Verification items for the finished model (mm, model axes). Face numbers are marked on the shaded views. A direction names the side the tool comes from. Give positions to 0.01 mm unless a question says otherwise; leave off trailing zeros. Order: outer loops, then holes, each group sorted by start corner. A loop starts at its lowest first (then second) coordinate and runs counter-clockwise, first axis right, second up.
from build123d import *

# Parameters (mm, degrees)
SKETCH1_W           = 30
SKETCH1_H           = 30
BOSS_EXTRUDE1_DEPTH = 7
SHELL1_T            = -1
SKETCH2_W           = 30
SKETCH2_H           = 7
BOSS_EXTRUDE2_DEPTH = 30
SKETCH3_W           = 30
SKETCH3_H           = 7
BOSS_EXTRUDE3_DEPTH = 30
SKETCH5_W           = 5
SKETCH5_H           = 23
BOSS_EXTRUDE4_DEPTH = 5
CUT_EXTRUDE6_DEPTH  = 23
SKETCH12_W          = 7.071067812
SKETCH12_H          = 23
BOSS_EXTRUDE6_DEPTH = 30
CUT_EXTRUDE7_DEPTH  = 22
CUT_EXTRUDE8_DEPTH  = 22
SHELL2_START        = 24
SHELL2_DEPTH        = 5
SHELL2_START_2      = 23
SHELL2_2_DEPTH      = 1
SHELL2_START_3      = 1
SHELL2_3_DEPTH      = 22
BOSS_EXTRUDE7_DEPTH = 1
BOSS_EXTRUDE8_DEPTH = 23
CUT_EXTRUDE10_DEPTH = 1
CUT_EXTRUDE12_START = -30
CUT_EXTRUDE12_DEPTH = 50


# Read off the part's stored shape, not the designer's step: Shell2
with BuildPart() as part:
    # Sketch1 → Boss-Extrude1 (new body)
    with BuildSketch(Plane.XY):
        with Locations((15, 15)):
            Rectangle(SKETCH1_W, SKETCH1_H)
    extrude(amount=BOSS_EXTRUDE1_DEPTH)

    # Shell1
    shell1_openings = [part.faces().sort_by_distance(p)[0] for p in [
        (30, 15, 3.5),
        (15, 0, 3.5),
    ]]
    offset(amount=SHELL1_T, openings=shell1_openings, kind=Kind.INTERSECTION)

    # Sketch2 → Boss-Extrude2 (add)
    with BuildSketch(Plane.XY.offset(7)):
        with Locations((15, 26.5)):
            Rectangle(SKETCH2_W, SKETCH2_H)
    extrude(amount=BOSS_EXTRUDE2_DEPTH)

    # Sketch3 → Boss-Extrude3 (add)
    with BuildSketch(Plane.ZY):
        with Locations((22, 26.5)):
            Rectangle(SKETCH3_W, SKETCH3_H)
    extrude(amount=BOSS_EXTRUDE3_DEPTH)

    # Sketch5 → Boss-Extrude4 (add)
    with BuildSketch(Plane.XY.offset(7)):
        with Locations((2.5, 11.5)):
            Rectangle(SKETCH5_W, SKETCH5_H)
    extrude(amount=BOSS_EXTRUDE4_DEPTH)

    # Sketch6 → Cut-Extrude6 (cut)
    with BuildSketch(Plane.XZ):
        Polygon((0, 12), (5, 12), (0, 7), align=None)
    extrude(amount=-CUT_EXTRUDE6_DEPTH, mode=Mode.SUBTRACT)

    # Sketch12 → Boss-Extrude6 (add)
    with BuildSketch(Plane(origin=(-3.5, 0, 3.5), x_dir=(0.7071067811865475, 0, 0.7071067811865477), z_dir=(-0.7071067811865477, 0, 0.7071067811865475))):
        with Locations((8.485281374, 11.5)):
            Rectangle(SKETCH12_W, SKETCH12_H)
    extrude(amount=BOSS_EXTRUDE6_DEPTH)

    # Sketch13 → Cut-Extrude7 (cut)
    with BuildSketch(Plane.XZ):
        Polygon((-19.798989873, 28.213203436), (0.707106781, 7.707106781), (4.292893219, 11.292893219), (-16.213203436, 31.798989873), (-16.920310217, 32.506096654), (-20.506096654, 28.920310217), align=None)
    extrude(amount=-CUT_EXTRUDE7_DEPTH, mode=Mode.SUBTRACT)

    # Sketch4 → Cut-Extrude8 (cut)
    with BuildSketch(Plane.XZ.offset(-23)):
        Polygon((-30, 37), (0, 7), (-30, 7), align=None)
    extrude(amount=-CUT_EXTRUDE8_DEPTH, mode=Mode.SUBTRACT)

    # Shell2 outline → Shell2 (cut)
    with BuildSketch(Plane(origin=(0, 0, 0), x_dir=(1, 0, 0), z_dir=(0, 1, 0)).offset(SHELL2_START)):
        Polygon((29, -37), (29, -7), (1, -7), (1, -7.414213562), (-28.585786438, -37), align=None)
    extrude(amount=SHELL2_DEPTH, mode=Mode.SUBTRACT)

    # Shell2 2 outline → Shell2 2 (cut)
    with BuildSketch(Plane(origin=(0, 0, 0), x_dir=(1, 0, 0), z_dir=(0, 1, 0)).offset(SHELL2_START_2)):
        Polygon((4, -7), (1, -7), (1, -7.414213562), (-19.798989873, -28.213203435), (-16.213203436, -31.798989873), (4, -11.585786438), align=None)
    extrude(amount=SHELL2_2_DEPTH, mode=Mode.SUBTRACT)

    # Shell2 3 outline → Shell2 3 (cut)
    with BuildSketch(Plane(origin=(0, 0, 0), x_dir=(1, 0, 0), z_dir=(0, 1, 0)).offset(SHELL2_START_3)):
        Polygon((4, -9.585786438), (4, -7), (1.414213562, -7), align=None)
    extrude(amount=SHELL2_3_DEPTH, mode=Mode.SUBTRACT)

    # Sketch16 → Boss-Extrude7 (add)
    with BuildSketch(Plane(origin=(0, 23, 0), x_dir=(1, 0, 0), z_dir=(0, 1, 0))):
        Polygon((1.414213562, -7), (1, -7), (1, -7.414213562), (-19.798989873, -28.213203436), (-16.213203436, -31.798989873), (4, -11.585786438), (4, -9.585786438), align=None)
    extrude(amount=BOSS_EXTRUDE7_DEPTH)

    # Sketch18 → Boss-Extrude8 (add)
    with BuildSketch(Plane(origin=(0, 1, 0), x_dir=(1, 0, 0), z_dir=(0, 1, 0))):
        Polygon((4, -9.585786438), (4, -7), (1.414213562, -7), align=None)
    extrude(amount=BOSS_EXTRUDE8_DEPTH)

    # Sketch19 → Cut-Extrude10 (cut)
    with BuildSketch(Plane(origin=(30, 0, 0), x_dir=(0, 0, -1), z_dir=(1, 0, 0))):
        Polygon((-36, 29), (-37, 29), (-37, 24), (-36, 24), (-7, 24), (-7, 29), align=None)
    extrude(amount=-CUT_EXTRUDE10_DEPTH, mode=Mode.SUBTRACT)

    # Mirror4: part across plane


with BuildPart() as part_1:
    add(part.part)
    add(part.part.mirror(Plane(origin=(0, 0, 7), x_dir=(0, 0, 1), z_dir=(0, 1, 0))))

    # Sketch20 → Cut-Extrude12 (cut)
    with BuildSketch(Plane.XZ.offset(30).offset(CUT_EXTRUDE12_START)):
        Polygon((0, 7), (0, 0), (30, 0), (30, 37), (-30, 37), align=None)
    extrude(amount=-CUT_EXTRUDE12_DEPTH, mode=Mode.SUBTRACT)


solid = part_1.part
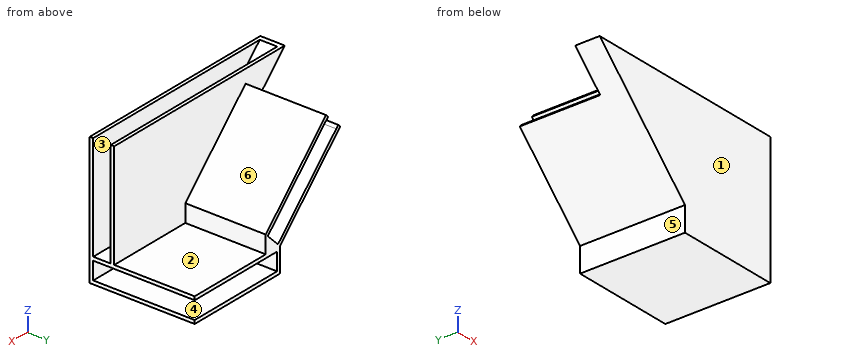
(1) Section check C-C, the plane z = 10. Enter the section's corners in (x, y), then the cut area to 3 significant figures.
Solved:
outline: (-3, -30) - (30, -30) - (30, -29) - (-1.59, -29) - (-1.59, -24) - (30, -24) - (30, -23) - (5, -23) - (5, 0) - (3, 0) - (3, -22) - (-1.59, -22) - (-1.59, 0) - (-3, 0) - close
area: 156 mm2
(2) Scan lines: line 1 (Z direction, x = 6, y = -28); line 2 (Y direction, x = 2, z = 34.5); line 3 (Z direction, x = 2, y = -10). Record each from-to range of solid material in increasing order.
Solved:
line 1: z = 0 to 1, 6 to 7
line 2: y = -30 to -29, -24 to -23
line 3: z = 0 to 1, 6 to 9, 13.59 to 15
(3) Go/stop test with flat-tipped pins: pin 1 (12 mm diameter, centred on x = -22, y = -5.5, fed in from +Z); pin 2 (4 mm diameter, centred on y = -22, z = 32.5, fed in from -X); pin 3 (2.5 mm diameter, centred on x = 16.5, y = -27.5, fed in from +Z). Record where each tip stops, or that it passes through.
Solved:
pin 1: stops at z = 33.21
pin 2: stops at x = -27.23
pin 3: stops at z = 7
(4) Release check for a two-part mould opening along Z. For the marked faces 4, 5 and 6 record: pulls with the +Z half, pulls with the -Z half, needs draft (parallel to the pull), parting line crosses it, or undercut.
Solved:
face 4: undercut
face 5: needs draft
face 6: pulls with the +Z half
(5) Section check D-D, the plane y = -3.25. Enter the section's corners in (x, z), then the cut area to 4 significant figures.
Solved:
outline: (-21.21, 28.21) - (0, 7) - (0, 0) - (30, 0) - (30, 1) - (1, 1) - (1, 6) - (30, 6) - (30, 7) - (5, 7) - (5, 12) - (-16.21, 33.21) - (-16.92, 32.51) - (4.29, 11.29) - (0.71, 7.71) - (-20.51, 28.92) - close
area: 137.5 mm2
(6) Section check B-B, the plane x = 15.5. Enter the section's corners in (y, z).
Solved:
outline: (-30, 0) - (0, 0) - (0, 1) - (-29, 1) - (-29, 6) - (0, 6) - (0, 7) - (-23, 7) - (-23, 37) - (-24, 37) - (-24, 7) - (-29, 7) - (-29, 37) - (-30, 37) - close
(7) Set-up check for the marked faces 1, 2 and 3: record each of +Z, -Z, +X, -X, +Y, -Y from which the full face is reachable in a straight line by a thin tool's end or side.
Solved:
face 1: +Z, -Z, +X, -X, -Y
face 2: +Z, +X, +Y
face 3: +Z, +X
(8) Section check A-A, the plane y = -27.25. Enter the section's corners in (x, z).
Solved:
outline: (-30, 37) - (0, 7) - (0, 0) - (30, 0) - (30, 1) - (1, 1) - (1, 6) - (30, 6) - (30, 7) - (1, 7) - (1, 7.41) - (-28.59, 37) - close
